Autodesk Inventor part; units mm, degrees
ref_plane "YZ Plane" through (0, 0, 0) normal (1, 0, 0) x (0, 1, 0)
ref_plane "XZ Plane" through (0, 0, 0) normal (0, 1, 0) x (-1, 0, 0)
ref_plane "XY Plane" through (0, 0, 0) normal (0, 0, 1) x (1, 0, 0)
sketch "Esquisse1" plane through (0, 0, 0) normal (0, 1, 0) x (-1, 0, 0)
  circle A0 centre (0, 0) radius 100
  line L0 (-10, -20) -> (10, -20)
  line L1 (10, -20) -> (10, 20)
  line L2 (10, 20) -> (-10, 20)
  line L3 (-10, 20) -> (-10, -20)
  line L4 (-10, -20) -> (10, 20) construction
  line L5 (10, -20) -> (-10, 20) construction
  dimension "d0" = 200
  dimension "d3" = 20
  dimension "d4" = 40
extrude "Extrusion2" add sketch "Esquisse1" along normal blind 8
sketch "Esquisse2" plane through (0, 0, 0) normal (0, -1, 0) x (1, 0, 0)
  line L0 (-55, -55) -> (55, -55)
  line L1 (55, -55) -> (55, 55)
  line L2 (55, 55) -> (-55, 55)
  line L3 (-55, 55) -> (-55, -55)
  line L4 (-55, -55) -> (55, 55) construction
  line L5 (55, -55) -> (-55, 55) construction
  circle A0 centre (-55, 55) radius 5
  circle A1 centre (55, 55) radius 5
  circle A2 centre (55, -55) radius 5
  circle A3 centre (-55, -55) radius 5
  point P0 (0, 0)
  dimension "d7" = 110
  dimension "d8" = 10
extrude "Extrusion3" cut sketch "Esquisse2" against normal blind 8 contours L3 A3 L0 | L0 A3 L3 | A2 L1 L0 | L0 L1 A2 | A0 L2 L3 | L3 L2 A0 | A1 L2 L1 | L1 L2 A1
properties part number "dessus" material "Bois (bouleau)"
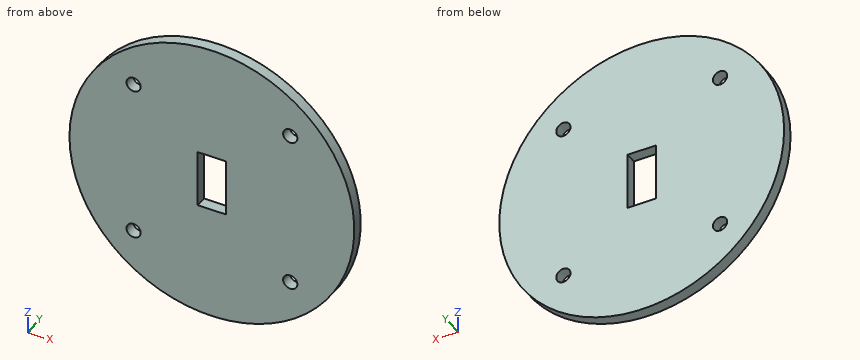
The model under review builds one solid part; all positions refer to its coordinate system, in mm. Round coordinates to 2 decimals unless told otherwise and drop trailing zeros. Order: outer loops, then holes, each group sorted by start corner. A loop starts at its lowest first (then second) coordinate and runs counter-clockwise, first axis right, second up. Notation, with made-up numbers: (-5, 72.25) -> (50, 72.25) arc R22 ccw to (50, 94.25) -> close; hole circle Ø10 at (-13, -16). An arc over 180 degrees is marked (long way). One line per item, written item: value. Start each with the question number.
Q1. Take a section at A-A (x = 0). Write out the cut boundary in (y, z).
Q2. Take a section at C-C (z = 55). Write out the cut boundary in (x, y), and give its area (3 significant figures).
Q3. Take a section at D-D (x = 55). Write out the cut boundary in (y, z).
Q4. Take a section at B-B (y = 2.5). Write out the cut boundary in (x, z).
Q5. Clearance check with flat-ended pins moving along their axes: pin 1 Ø2.5 at (x, y) = (-4, 3) entering from +Z; pin 2 Ø2.5 at (y, z) = (5, 7) entering from -X; pin 3 Ø3 at (x, y) = (-7, 4) entering from +Z. State where each tip first meets the part, or that it passes through.
Q6. Wall thickness on line 1 (X direction, y = 2.75, z = -55); line 2 (Z direction, x = 59, y = 4.75): over which ranges is each line inside the solid? List them lowest first.
Reported:
1. outline: (0, -100) -> (8, -100) -> (8, -20) -> (0, -20) -> close; (0, 20) -> (8, 20) -> (8, 100) -> (0, 100) -> close
2. outline: (-83.52, 0) -> (-60, 0) -> (-60, 8) -> (-83.52, 8) -> close; (-50, 0) -> (50, 0) -> (50, 8) -> (-50, 8) -> close; (60, 0) -> (83.52, 0) -> (83.52, 8) -> (60, 8) -> close
2. area: 1,180 mm2
3. outline: (0, -83.52) -> (8, -83.52) -> (8, -60) -> (0, -60) -> close; (0, -50) -> (8, -50) -> (8, 50) -> (0, 50) -> close; (0, 60) -> (8, 60) -> (8, 83.52) -> (0, 83.52) -> close
4. outline: circle Ø200 at (0, 0); hole circle Ø10 at (-55, -55); hole circle Ø10 at (-55, 55); hole (-10, -20) -> (10, -20) -> (10, 20) -> (-10, 20) -> close; hole circle Ø10 at (55, -55); hole circle Ø10 at (55, 55)
5. pin 1: stops at z = 99.96
5. pin 2: stops at x = -99.83
5. pin 3: stops at z = 99.85
6. line 1: x = -83.52 to -60, -50 to 50, 60 to 83.52
6. line 2: z = -80.74 to -58, -52 to 52, 58 to 80.74
